Can you work these out from the model? Positions are in its coordinate system, mm. Face numbers are marked on the shaded views. Coordinates: 2 decimals unless noted, no trailing zeros. Order: outer loops, then holes, each group sorted by start corner. A loop starts at its lowest first (then second) coordinate and runs counter-clockwise, first axis right, second up. Notation, with made-up numbers: (-24, -3.5) - (6, -3.5) arc R8 cw to (6, 7.5) - close; hole circle Ø5 at (89, 44). An arc over 180 degrees is marked (long way). Return JSON: item names as keys, results as strings. Group by question number.
1) Imagine slicing it at B-B (z = 15.75). Write out the boundary of the cut face in (x, y) (1 decimal), and give its area (3 significant figures).
2) Imagine slicing it at C-C (x = 0). Write out the boundary of the cut face in (y, z).
3) For pin 1 Ø3 at (y, z) = (3.5, 17) entering from -X; pin 2 Ø0.7 at (y, z) = (-0.5, 2.5) entering from +X; pin 3 Ø2.5 at (x, y) = (0, 0) entering from +Z, each with a flat end and sliding along its axis, tell me the tip position at first contact or that it passes through.
4) Imagine slicing it at A-A (y = 0). Write out the boundary of the cut face in (x, z), and give its area (3 significant figures).
5) If I drill on line 1 along Y through (x, z) = (0, 6.5); line 2 along Y through (x, z) = (1.5, 19); line 3 along Z through (x, y) = (0, -0.75), over which ranges is the centre line in solid material (lowest first)?
6) Imagine slicing it at D-D (x = -1.25). Write out the boundary of the cut face in (y, z), and give its area (3 significant figures).
7) If we mould it in two halves opening along Y, with no side actions, what happens to the marked faces 1, 2 and 3? For each: pulls with the +Y half, pulls with the -Y half, needs draft (parallel to the pull), parting line crosses it, or undercut.
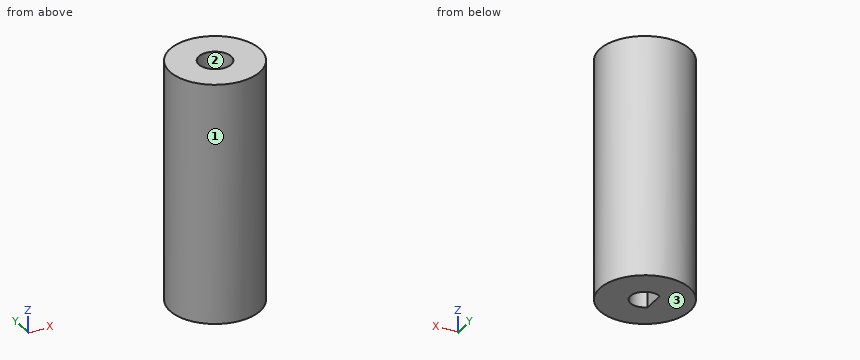
Autodesk Inventor part; units mm, degrees
ref_plane "YZ Plane" through (0, 0, 0) normal (1, 0, 0) x (0, 1, 0)
ref_plane "XZ Plane" through (0, 0, 0) normal (0, 1, 0) x (-1, 0, 0)
ref_plane "XY Plane" through (0, 0, 0) normal (0, 0, 1) x (1, 0, 0)
sketch "Sketch1" plane through (0, 0, 0) normal (0, 0, 1) x (1, 0, 0)
  arc A0 (-0.9144, -1.2192) -> (-0.9144, 1.2192) centre (0, 0) ccw
  line L0 (-0.9144, 1.2192) -> (-0.9144, -1.2192)
  circle A1 centre (0, 0) radius 4.7625
  point P0 (-0.889, 0)
  point P1 (1.524, 0)
  dimension "d0" = 3.048
  dimension "d2" = 2.413
  dimension "d3" = 9.525
extrude "Extrusion1" add sketch "Sketch1" along normal blind 10.16
sketch "Sketch2" plane through (0, 0, 10.16) normal (0, 0, 1) x (1, 0, 0)
  circle A0 centre (0, 0) radius 4.7625
extrude "Extrusion2" add sketch "Sketch2" along normal blind 6.35
sketch "Sketch3" plane through (0, 0, 16.51) normal (0, 0, 1) x (1, 0, 0)
  circle A0 centre (0, 0) radius 4.7625
  circle A1 centre (0, 0) radius 1.7145
  dimension "d8" = 3.429
extrude "Extrusion3" add sketch "Sketch3" along normal blind 12.7
sketch "Sketch4" plane through (0, 0, 29.21) normal (0, 0, 1) x (1, 0, 0)
  circle A0 centre (0, 0) radius 1.7145
  circle A1 centre (0, 0) radius 4.7625
extrude "Extrusion4" cut sketch "Sketch4" against normal blind 3.81
sketch "Sketch5" plane through (0, 0, 16.51) normal (0, 0, 1) x (1, 0, 0)
  circle A0 centre (0, 0) radius 1.7145
extrude "Extrusion5" cut sketch "Sketch5" against normal blind 3.81
properties part number "Coupling Bushing" material "ABS Plastic"
Calculated:
{
 "1": {"outline": "circle Ø9.5 at (0, 0); hole circle Ø3.4 at (0, 0)", "area": "62.0 mm2"},
 "2": {"outline": "(-4.76, 0) - (-1.52, 0) - (-1.52, 10.16) - (1.52, 10.16) - (1.52, 0) - (4.76, 0) - (4.76, 25.4) - (1.71, 25.4) - (1.71, 12.7) - (-1.71, 12.7) - (-1.71, 25.4) - (-4.76, 25.4) - close"},
 "3": {"pin 1": "x = -4.32", "pin 2": "x = 4.76", "pin 3": "z = 12.7"},
 "4": {"outline": "(-4.76, 0) - (-0.91, 0) - (-0.91, 10.16) - (1.52, 10.16) - (1.52, 0) - (4.76, 0) - (4.76, 25.4) - (1.71, 25.4) - (1.71, 12.7) - (-1.71, 12.7) - (-1.71, 25.4) - (-4.76, 25.4) - close", "area": "174 mm2"},
 "5": {"line 1": "-4.76 to -1.52, 1.52 to 4.76", "line 2": "-4.52 to -0.83, 0.83 to 4.52", "line 3": "10.16 to 12.7"},
 "6": {"outline": "(-4.6, 0) - (4.6, 0) - (4.6, 25.4) - (1.17, 25.4) - (1.17, 12.7) - (-1.17, 12.7) - (-1.17, 25.4) - (-4.6, 25.4) - close", "area": "204 mm2"},
 "7": {"face 1": "parting line crosses it", "face 2": "undercut", "face 3": "needs draft"}
}
